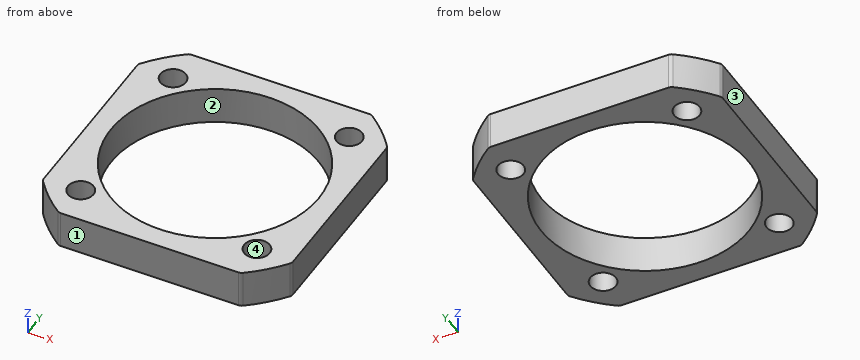
Autodesk Inventor part; units mm, degrees
ref_plane "YZ Plane" through (0, 0, 0) normal (1, 0, 0) x (0, 1, 0)
ref_plane "XZ Plane" through (0, 0, 0) normal (0, 1, 0) x (-1, 0, 0)
ref_plane "XY Plane" through (0, 0, 0) normal (0, 0, 1) x (1, 0, 0)
sketch "Sketch1" plane through (0, 0, 0) normal (0, 0, 1) x (1, 0, 0)
  line L0 (21, -21) -> (-21, -21)
  line L1 (-21, -21) -> (-21, 21)
  line L2 (-21, 21) -> (21, 21)
  line L3 (21, 21) -> (21, -21)
  line L4 (21, -21) -> (-21, 21) construction
  line L5 (-21, -21) -> (21, 21) construction
  circle A0 centre (0, 0) radius 17.5
  circle A1 centre (0, 0) radius 26
  line L6 (0, 0) -> (-9.5671, 23.097) construction
  line L7 (0, 0) -> (0, 21) construction
  point P0 (-15.3297, 21)
  point P1 (-21, 15.3297)
  point P2 (-21, -15.3297)
  point P3 (-15.3297, -21)
  point P4 (15.3297, -21)
  point P5 (21, -15.3297)
  point P6 (21, 15.3297)
  point P7 (15.3297, 21)
  dimension "d0" = 42
  dimension "d1" = 42
  dimension "d2" = 35
  dimension "d3" = 52
  dimension "d4" = 25
  dimension "d5" = 22.5
extrude "Extrusion1" add sketch "Sketch1" along normal blind 6.35 contours L0 A1 L1 L2 L3
sketch "Sketch2" plane through (0, 0, 6.35) normal (0, 0, 1) x (1, 0, 0)
  line L0 (14.8492, -14.8492) -> (-14.8492, -14.8492)
  line L1 (-14.8492, -14.8492) -> (-14.8492, 14.8492)
  line L2 (-14.8492, 14.8492) -> (14.8492, 14.8492)
  line L3 (14.8492, 14.8492) -> (14.8492, -14.8492)
  line L4 (14.8492, -14.8492) -> (-14.8492, 14.8492) construction
  line L5 (-14.8492, -14.8492) -> (14.8492, 14.8492) construction
  point P0 (0, 0)
  dimension "d20" = 42
hole "Hole2" at (-14.8492, 14.8492, 6.35) at (14.8492, 14.8492, 6.35) at (14.8492, -14.8492, 6.35) at (-14.8492, -14.8492, 6.35) direction (0, 0, -1) diameter 4.3 end through all
fillet "Fillet1" radius 1 8 edges at (15.3297, -21, 3.175) (21, -15.3297, 3.175) (-21, -15.3297, 3.175) (-15.3297, -21, 3.175) (21, 15.3297, 3.175) (15.3297, 21, 3.175) (-21, 15.3297, 3.175) (-15.3297, 21, 3.175)
properties part number "Ballscrew Spacer"
Geometry: final body of the model. Coordinates: model frame, mm. Face numbers are marked on the shaded views. Give positions to 0.01 mm unless a question says otherwise; leave off trailing zeros. Write each loop counter-clockwise with the first axis right and the second up, starting at its lowest first coordinate (ties: lowest second). Pieces come first, ordered by that corner, then holes. Notation, with made-up numbers: (31, 8) - (43, 8) arc R24 ccw to (43, 24) - close; hole circle Ø6 at (-9.75, 17.5). An arc over 180 degrees is marked (long way). Return JSON: item names as keys, results as strings. Group by question number.
1) Mould query, pull axis X, two halves, no side actions, for the marked faces 1, 2, 3 and 4. Classes: released by +X, released by -X, zero draft, split by the parting line, or undercut.
2) Section A-A on x = 0. Return the cut outline in (y, z), plus the area to 4 significant figures.
3) Section C-C on y = -14. Return the cut outline in (x, z), plus the area to 3 significant figures.
4) Line query: line 1 (Y direction, x = -14.5, z = 4.5); line 2 (Y direction, x = 13, z = 3.25); line 3 (Y direction, x = 9, z = 3.75). Output: solid intervals per line, ascending.
Filled in:
{
 "1": {"face 1": "zero draft", "face 2": "undercut", "face 3": "released by -X", "face 4": "undercut"},
 "2": {"outline": "(-21, 0) - (-17.5, 0) - (-17.5, 6.35) - (-21, 6.35) - close; (17.5, 0) - (21, 0) - (21, 6.35) - (17.5, 6.35) - close", "area": "44.45 mm^2"},
 "3": {"outline": "(-21, 0) - (-16.82, 0) - (-16.82, 6.35) - (-21, 6.35) - close; (-12.87, 0) - (-10.5, 0) - (-10.5, 6.35) - (-12.87, 6.35) - close; (10.5, 0) - (12.87, 0) - (12.87, 6.35) - (10.5, 6.35) - close; (16.82, 0) - (21, 0) - (21, 6.35) - (16.82, 6.35) - close", "area": "83.2 mm^2"},
 "4": {"line 1": "y = -21 to -16.97, -12.73 to -9.8, 9.8 to 12.73, 16.97 to 21", "line 2": "y = -21 to -15.95, -13.75 to -11.72, 11.72 to 13.75, 15.95 to 21", "line 3": "y = -21 to -15.01, 15.01 to 21"}
}
